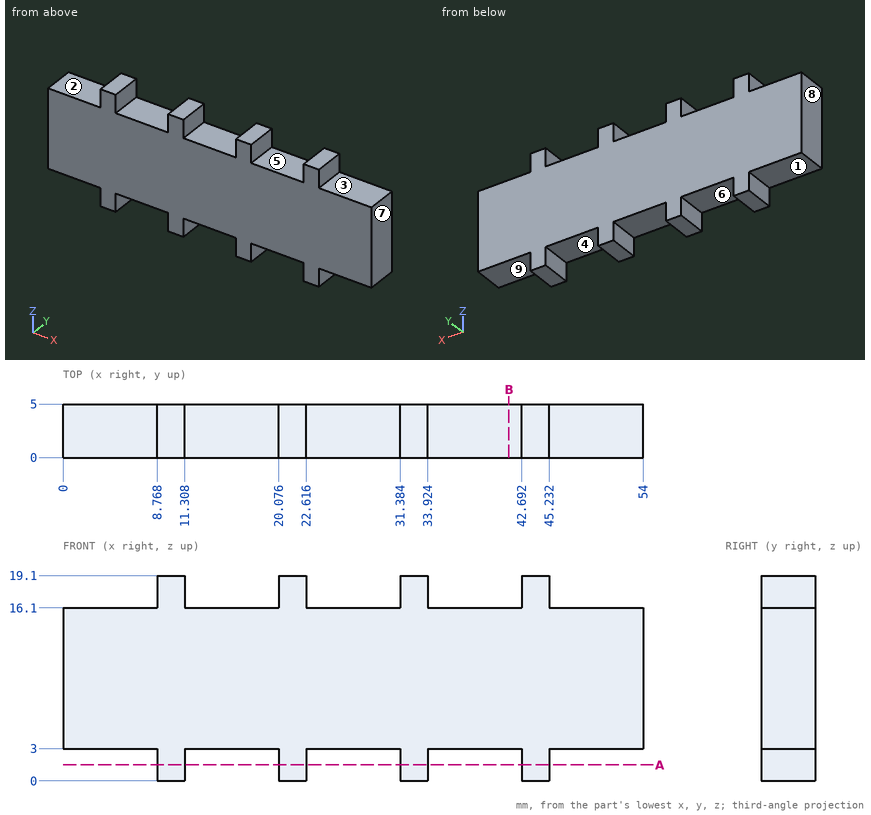
Study the drawing (mm; zero at the part's minimum x, y, z) and answer. A direction names the side the tool comes from. Round coordinates to 2 decimals unless told otherwise and drop trailing zeros. Order: outer loops, then holes, each group sorted by start corner. A loop starts at its lowest first (then second) coordinate and runs counter-clockwise, first axis right, second up. Notation, with made-up numbers: (0.25, 8) - (56.25, 8) arc R33 cw to (56.25, 38) - close; hole circle Ø3 at (79, 68). An arc over 180 degrees is marked (long way). Use one line per item in the form item = value. Start each with the question number.
(1) For the marked faces 1, 2, 3, 4 and 5, determine the directions among +Z, -Z, +X, -X, +Y, -Y from which every point of the face is accessible in a straight line to the end or side of a thin tool.
(2) Determine the mould class of the marked faces 6, 7, 8 and 9 for opening direction X: +X half, -X half, draft (parallel to the pull), parting line (faces both ways), or undercut.
(3) The part is cut by section B-B (x = 41.5). Give the vertices of the cut face in (y, z).
(4) Find the intervals of material crossed by line 1 along X through (y, z) = (3.3, 18); line 2 along Z through (x, y) = (29, 4.65), in increasing order. Write a range as from..to.
(5) Flat-ended cylindrical pins translate along their axes: pin 1 Ø0.9 at (y, z) = (3, 1) entering from -X; pin 2 Ø1.5 at (y, z) = (2, 1) entering from +X; pin 3 Ø1.5 at (x, y) = (29, 3) entering from -Z; pin 4 Ø6 at (x, z) = (46, 6) entering from -Y. Find the tip coordinate at first contact, or state that the pin passes through.
(6) The part is cut by section A-A (z = 1.5). Give the vertices of the cut face in (x, y), then the cut area to 3 significant figures.
Checked values:
q1.face_1 = -Z, -X, +Y, -Y
q1.face_2 = +Z, -X, +Y, -Y
q1.face_3 = +Z, +X, +Y, -Y
q1.face_4 = -Z, +Y, -Y
q1.face_5 = +Z, +Y, -Y
q2.face_6 = undercut
q2.face_7 = +X half
q2.face_8 = -X half
q2.face_9 = draft
q3.outline = (0, 3) - (5, 3) - (5, 16.1) - (0, 16.1) - close
q4.line_1 = 8.77..11.31, 20.08..22.62, 31.38..33.92, 42.69..45.23
q4.line_2 = 3..16.1
q5.pin_1 = 8.77
q5.pin_2 = 45.23
q5.pin_3 = 3
q5.pin_4 = 0
q6.outline = (8.77, 0) - (11.31, 0) - (11.31, 5) - (8.77, 5) - close; (20.08, 0) - (22.62, 0) - (22.62, 5) - (20.08, 5) - close; (31.38, 0) - (33.92, 0) - (33.92, 5) - (31.38, 5) - close; (42.69, 0) - (45.23, 0) - (45.23, 5) - (42.69, 5) - close
q6.area = 50.8 mm^2
